Here's how the part is built. I have some questions about the finished solid (model axes, mm). Face numbers are marked on the shaded views. A direction names the side the tool comes from. Coordinates: 2 decimals unless noted, no trailing zeros. Write each loop counter-clockwise with the first axis right and the second up, starting at its lowest first coordinate (ties: lowest second). Pieces come first, ordered by that corner, then holes.
(1) Please list where these lines run through material, in increasing order: probe 1 along Z at (x, y) = (0, -5.25); probe 2 along Y at (x, z) = (1.5, 15); probe 3 along X at (y, z) = (-3.75, -14.5).
(2) Imagine slicing it at B-B, the plane z = 0. List the corners of the cut face in (x, y) for me.
(3) Imagine slicing it at C-C, the plane y = -23.75. List the corners of the cut face in (x, z) for me, plus the area to 3 significant figures.
(4) Which directions (+Z, -Z, +X, -X, +Y, -Y) give clear straight access to the entire face, cutting with the end or side of a thin tool? Please do the marked faces 1 and 2.
(5) For pin 1 Ø4 at (y, z) = (-5.5, 2) entering from +X; pin 2 Ø5 at (y, z) = (-22, 10.5) entering from +X; pin 3 Ø6 at (x, z) = (10, -9) entering from +Y, each with a flat end and sliding along its axis, tell me the tip position at first contact or that it passes through.
(6) Imagine slicing it at A-A, the plane x = 0. List the corners of the cut face in (y, z) for me, plus the area to 3 significant figures.
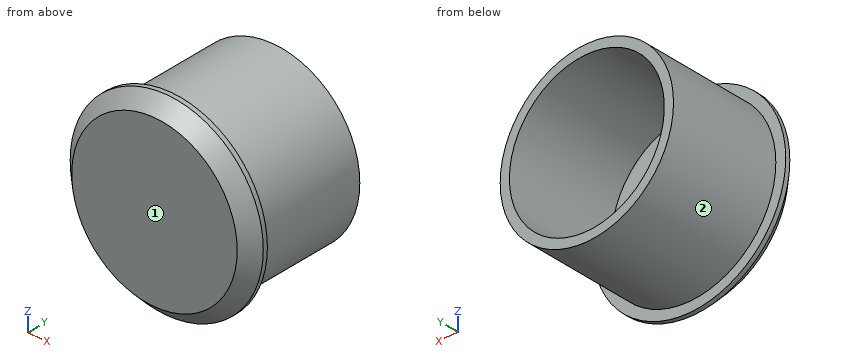
```python
from build123d import *

# Parameters (mm, degrees)
F0_R     = 18.85
F0_R_2   = 16.85
F1_DEPTH = 25
F2_R     = 21
F3_DEPTH = 4
F4_SIZE  = 3


with BuildPart() as f1:
    # F0 (on Front) → F1 (new body)
    with BuildSketch(Plane.XZ):
        Circle(F0_R)
        Circle(F0_R_2, mode=Mode.SUBTRACT)
    extrude(amount=F1_DEPTH)

    # F2 (on face) → F3 (join)
    with BuildSketch(Plane.XZ.offset(25)):
        Circle(F2_R)
    extrude(amount=F3_DEPTH)

    # F4
    f4_edges = [f1.edges().sort_by_distance(p)[0] for p in [
        (-21, -29, 0),
    ]]
    chamfer(f4_edges, length=F4_SIZE)


solid = f1.part
```
Recorded:
1. probe 1: z = -18.85 to -16.85, 16.85 to 18.85
1. probe 2: y = -29 to -25
1. probe 3: x = -12.04 to -8.58, 8.58 to 12.04
2. outline: (-21, -26) - (-18, -29) - (18, -29) - (21, -26) - (21, -25) - (18.85, -25) - (18.85, 0) - (16.85, 0) - (16.85, -25) - (-16.85, -25) - (-16.85, 0) - (-18.85, 0) - (-18.85, -25) - (-21, -25) - close
3. outline: circle Ø37.7 at (0, 0); hole circle Ø33.7 at (0, 0)
3. area: 224 mm2
4. face 1: +Z, -Z, +X, -X, -Y
4. face 2: +Y
5. pin 1: stops at x = 18.85
5. pin 2: stops at x = 17.07
5. pin 3: stops at y = -25
6. outline: (-29, -18) - (-26, -21) - (-25, -21) - (-25, -18.85) - (0, -18.85) - (0, -16.85) - (-25, -16.85) - (-25, 16.85) - (0, 16.85) - (0, 18.85) - (-25, 18.85) - (-25, 21) - (-26, 21) - (-29, 18) - close
6. area: 259 mm2
